Build history of the part. All positions in model axes, mm. A direction names the side the tool comes from. Give positions to 0.01 mm unless a question says otherwise; leave off trailing zeros. Loops run counter-clockwise (first coordinate to the right, second up) from the corner with the lowest first, then second, coordinate; pieces in that order, holes last. Notation, with made-up numbers: (55.5, -6.75) - (72.5, -6.75) arc R26 ccw to (72.5, 7.25) - close; hole circle Ø10 at (-32.75, -10.75). An arc over 180 degrees is marked (long way). Return JSON: item names as keys, results as strings. Group by question number.
1) Slice it at D-D (y = 18.5). List the corners of the cut face in (x, z).
2) Slice it at C-C (z = -6). List the corners of the cut face in (x, y), and give its area (3 significant figures).
3) 3-axis set-ups, long thin cutter, end or side, ignore diameter. For faces 4 (the face through (6.604, 37, -6)), 5 (the face through (12, 30, 24.892)), 6 (the face through (17.272, 37, -6)), 7 (the face through (32.627, 11.301, -7.405)), 8 (the face through (-9.77, 20.12, -15.79)): which of +Z, -Z, +X, -X, +Y, -Y reach the whole face in a straight line?
4) Drop flat-ended pins along their axis: pin 1 (2.5 mm diameter, centred on x = 19.63, z = -3.23, fed in from +Y); pin 2 (5 mm diameter, centred on x = 14.5, z = 6.5, fed in from -Y); pin 3 (5.5 mm diameter, centred on x = 3, z = -30, fed in from +Y); pin 4 (0.8 mm diameter, centred on x = 13, z = 26.5, fed in from +Y). Give the stop position or say it passes through.
5) Mould opens along Z. For faces 1 (the face through (11, 0, -21)), 2 (the face through (32.63, 8.92, -32.37)), 3 (the face through (12, 46, 24.892)) say: released by +Z, released by -Z, zero draft, split by the parting line, or undercut.
6) Slice it at B-B (x = 11.5). List the corners of the cut face in (y, z).
7) Slice it at A-A (y = 11). List the corners of the cut face in (x, z).
8) Drill centre lines: probe 1 along X at (y, z) = (47.5, 1.5); probe 2 along X at (y, z) = (23, -1); probe 3 along Y at (x, z) = (1, -20.5). Where is each one in solid material? Low to high. Write a range as from..to.
```python
from build123d import *

# Parameters (mm, degrees)
SKETCH1_W           = 22.86
SKETCH1_H           = 41.148
BOSS_EXTRUDE1_DEPTH = 23.368
SKETCH2_W           = 10.668
SKETCH2_H           = 66.04
BOSS_EXTRUDE2_DEPTH = 27.94
SKETCH3_R           = 6.35
BOSS_EXTRUDE3_DEPTH = 19.812
SKETCH4_R           = 6.35
BOSS_EXTRUDE4_DEPTH = 19.812
SKETCH5_W           = 10.668
SKETCH5_H           = 3.048
BOSS_EXTRUDE5_DEPTH = 2.54
SKETCH6_R           = 1.7145
CUT_EXTRUDE1_DEPTH  = 79.400053265


with BuildPart() as part:
    # Sketch1 → Boss-Extrude1 (new body)
    with BuildSketch(Plane(origin=(0, 0, 0), x_dir=(1, 0, 0), z_dir=(0, 1, 0))):
        with Locations((11.43, 20.574)):
            Rectangle(SKETCH1_W, SKETCH1_H)
    extrude(amount=BOSS_EXTRUDE1_DEPTH)

    # Sketch2 → Boss-Extrude2 (add)
    with BuildSketch(Plane(origin=(0, 23.368, 0), x_dir=(1, 0, 0), z_dir=(0, 1, 0))):
        with Locations((11.938, 8.128)):
            Rectangle(SKETCH2_W, SKETCH2_H)
    extrude(amount=BOSS_EXTRUDE2_DEPTH)

    # Sketch3 → Boss-Extrude3 (add)
    with BuildSketch(Plane.ZY):
        with Locations(Location((-20.828, 16.256, 0), (0, 0, 180))):
            Circle(SKETCH3_R)
    extrude(amount=BOSS_EXTRUDE3_DEPTH)

    # Sketch4 → Boss-Extrude4 (add)
    with BuildSketch(Plane(origin=(22.86, 0, 0), x_dir=(0, 0, -1), z_dir=(1, 0, 0))):
        with Locations(Location((27.686, 13.208, 0), (0, 0, 180))):
            Circle(SKETCH4_R)
        with Locations(Location((13.462, 13.208, 0), (0, 0, 180))):
            Circle(SKETCH4_R)
    extrude(amount=BOSS_EXTRUDE4_DEPTH)

    # Sketch5 → Boss-Extrude5 (add)
    with BuildSketch(Plane.XY.offset(24.892)):
        with Locations((11.938, 39.116)):
            Rectangle(SKETCH5_W, SKETCH5_H)
    extrude(amount=BOSS_EXTRUDE5_DEPTH)

    # Sketch6 → Cut-Extrude1 (cut, through all)
    with BuildSketch(Plane(origin=(0, 0, 0), x_dir=(-1, 0, 0), z_dir=(0, -1, 0))):
        with Locations(Location((-19.6342, 3.2258, 0), (0, 0, 90))):
            Circle(SKETCH6_R)
        with Locations(Location((-19.6342, 37.9222, 0), (0, 0, 90))):
            Circle(SKETCH6_R)
    extrude(amount=-CUT_EXTRUDE1_DEPTH, mode=Mode.SUBTRACT)


solid = part.part
```
Results:
{
 "1": {"outline": "(-19.81, -26.77) - (0, -26.77) - (0, -41.15) - (22.86, -41.15) - (22.86, -31.2) - (42.67, -31.2) - (42.67, -24.18) - (22.86, -24.18) - (22.86, -16.97) - (42.67, -16.97) - (42.67, -9.95) - (22.86, -9.95) - (22.86, 0) - (0, 0) - (0, -14.89) - (-19.81, -14.89) - close; hole circle Ø3.43 at (19.63, -37.92); hole circle Ø3.43 at (19.63, -3.23)"},
 "2": {"outline": "(0, 0) - (22.86, 0) - (22.86, 23.37) - (17.27, 23.37) - (17.27, 51.31) - (6.6, 51.31) - (6.6, 23.37) - (0, 23.37) - close", "area": "832 mm2"},
 "3": {"face 4": "+Z, -Z, -X, +Y", "face 5": "+Z, +X, -X, -Y", "face 6": "+Z, -Z, +X, +Y", "face 7": "+X", "face 8": "-X"},
 "4": {"pin 1": "through", "pin 2": "y = 23.37", "pin 3": "y = 23.37", "pin 4": "y = 40.64"},
 "5": {"face 1": "zero draft", "face 2": "undercut", "face 3": "released by +Z"},
 "6": {"outline": "(0, -41.15) - (51.31, -41.15) - (51.31, 24.89) - (40.64, 24.89) - (40.64, 27.43) - (37.59, 27.43) - (37.59, 24.89) - (23.37, 24.89) - (23.37, 0) - (0, 0) - close"},
 "7": {"outline": "(-19.81, -24.39) - (0, -24.39) - (0, -41.15) - (22.86, -41.15) - (22.86, -33.64) - (42.67, -33.64) - (42.67, -21.73) - (22.86, -21.73) - (22.86, -19.42) - (42.67, -19.42) - (42.67, -7.51) - (22.86, -7.51) - (22.86, 0) - (0, 0) - (0, -17.26) - (-19.81, -17.26) - close; hole circle Ø3.43 at (19.63, -37.92); hole circle Ø3.43 at (19.63, -3.23)"},
 "8": {"probe 1": "6.6..17.27", "probe 2": "0..22.86", "probe 3": "0..23.37"}
}
